```python
from build123d import *

# Parameters (mm, degrees)
CYLINDER412_R               = 1.5
CYLINDER412_DEPTH           = 60
CYLINDER410_R               = 1.5
CYLINDER410_DEPTH           = 60
CYLINDER410_PLACEMENT_ANGLE = 135
CYLINDER408_R               = 1.5
CYLINDER408_DEPTH           = 60
CYLINDER411_R               = 1.5
CYLINDER411_DEPTH           = 60
CYLINDER411_PLACEMENT_ANGLE = 225
CYLINDER414_R               = 1.5
CYLINDER414_DEPTH           = 60
CYLINDER407_R               = 1.5
CYLINDER407_DEPTH           = 60
CYLINDER407_PLACEMENT_ANGLE = 45
CYLINDER413_R               = 1.5
CYLINDER413_DEPTH           = 60
CYLINDER409_R               = 1.5
CYLINDER409_DEPTH           = 60
CYLINDER409_PLACEMENT_ANGLE = 45
COMPOUND307_PLACEMENT_ANGLE = 22.5
TUBE036_R                   = 46
TUBE036_R_2                 = 38
TUBE036_DEPTH               = 3


with BuildPart() as obj1:
    # Cylinder412 → Cylinder412 (new body)
    with BuildSketch(Plane(origin=(0, 41, -54), x_dir=(0, 1, 0), z_dir=(0, 0, 1))):
        Circle(CYLINDER412_R)
    extrude(amount=CYLINDER412_DEPTH)


with BuildPart() as obj2:
    # Cylinder410 → Cylinder410 (new body)
    with BuildSketch(Plane.XY):
        Circle(CYLINDER410_R)
    extrude(amount=CYLINDER410_DEPTH)


with BuildPart() as obj2_1:
    # Cylinder410 placement: moved
    add(obj2.part.moved(Location((-28.991378, 28.991378, -54))).rotate(Axis((-28.991378, 28.991378, -54), (0, 0, 1)), CYLINDER410_PLACEMENT_ANGLE))


with BuildPart() as obj3:
    # Cylinder408 → Cylinder408 (new body)
    with BuildSketch(Plane(origin=(-41, 0, -54), x_dir=(-1, 0, 0), z_dir=(0, 0, 1))):
        Circle(CYLINDER408_R)
    extrude(amount=CYLINDER408_DEPTH)


with BuildPart() as obj4:
    # Cylinder411 → Cylinder411 (new body)
    with BuildSketch(Plane.XY):
        Circle(CYLINDER411_R)
    extrude(amount=CYLINDER411_DEPTH)


with BuildPart() as obj4_1:
    # Cylinder411 placement: moved
    add(obj4.part.moved(Location((-28.991378, -28.991378, -54))).rotate(Axis((-28.991378, -28.991378, -54), (0, 0, 1)), CYLINDER411_PLACEMENT_ANGLE))


with BuildPart() as obj5:
    # Cylinder414 → Cylinder414 (new body)
    with BuildSketch(Plane(origin=(0, -41, -54), x_dir=(0, -1, 0), z_dir=(0, 0, 1))):
        Circle(CYLINDER414_R)
    extrude(amount=CYLINDER414_DEPTH)


with BuildPart() as obj6:
    # Cylinder407 → Cylinder407 (new body)
    with BuildSketch(Plane.XY):
        Circle(CYLINDER407_R)
    extrude(amount=CYLINDER407_DEPTH)


with BuildPart() as obj6_1:
    # Cylinder407 placement: moved
    add(obj6.part.moved(Location((28.991378, -28.991378, -54))).rotate(Axis((28.991378, -28.991378, -54), (0, 0, -1)), CYLINDER407_PLACEMENT_ANGLE))


with BuildPart() as obj7:
    # Cylinder413 → Cylinder413 (new body)
    with BuildSketch(Plane(origin=(41, 0, -54), x_dir=(1, 0, 0), z_dir=(0, 0, 1))):
        Circle(CYLINDER413_R)
    extrude(amount=CYLINDER413_DEPTH)


with BuildPart() as compound307:
    # Cylinder409 → Cylinder409 (new body)
    with BuildSketch(Plane.XY):
        Circle(CYLINDER409_R)
    extrude(amount=CYLINDER409_DEPTH)


with BuildPart() as compound307_1:
    # Cylinder409 placement: moved
    add(compound307.part.moved(Location((28.991378, 28.991378, -54))).rotate(Axis((28.991378, 28.991378, -54), (0, 0, 1)), CYLINDER409_PLACEMENT_ANGLE))

    # Compound307: union obj1, obj2, obj3, obj4, obj5, obj6, obj7
    add(obj1.part)
    add(obj2_1.part)
    add(obj3.part)
    add(obj4_1.part)
    add(obj5.part)
    add(obj6_1.part)
    add(obj7.part)


with BuildPart() as compound307_2:
    # Compound307 placement: moved
    add(compound307_1.part.rotate(Axis((0, 0, 0), (0, 0, 1)), COMPOUND307_PLACEMENT_ANGLE))


with BuildPart() as j_midi_motor_washer:
    # Tube036 → Tube036 (new body)
    with BuildSketch(Plane.XY.offset(-11)):
        Circle(TUBE036_R)
        Circle(TUBE036_R_2, mode=Mode.SUBTRACT)
    extrude(amount=TUBE036_DEPTH)

    # Cut162: cut Compound307
    add(compound307_2.part, mode=Mode.SUBTRACT)


solid = j_midi_motor_washer.part
```
Work out the finished part from the listing and answer in its coordinate system (mm). Coordinates: 2 decimals unless noted, no trailing zeros. Loops run counter-clockwise (first coordinate to the right, second up) from the corner with the lowest first, then second, coordinate; pieces in that order, holes last.
1) Section A-A (y = 0) is taken. Give the vertices of the cut face in (x, z), plus the area to 3 significant figures.
Results:
outline: (-46, -11) - (-38, -11) - (-38, -8) - (-46, -8) - close; (38, -11) - (46, -11) - (46, -8) - (38, -8) - close
area: 48.0 mm2
2) Consider probe 1 along X at (y, z) = (1, -9.6); probe 2 along Y at (x, z) = (13, -9.85); probe 3 along Y at (x, z) = (-23, -9.15). Determine where each line is inside the solid, lowest interval first.
Results:
probe 1: x = -45.99 to -37.99, 37.99 to 45.99
probe 2: y = -44.12 to -35.71, 35.71 to 44.12
probe 3: y = -39.84 to -30.25, 30.25 to 39.84
3) A flat-ended cylindrical pin translates along its axis: pin 1 (4 mm diameter, centred on x = 15.69, y = -37.88, fed in from -Z). Find the tip coordinate at first contact, or state that the pin passes through.
Results:
pin 1: stops at z = -11
4) Section C-C (z = -8.75) is taken. Give the number of separate pieces and of enclosed holes in the cut face, plus the area to 3 significant figures.
Results:
separate pieces: 1
enclosed holes: 9
area: 2,050 mm2
5) For a pull along Y with two mould halves and no side action, classify faces 1 (the cylindrical face through (-5.99, 45.61, -9.52)), 2 (the cylindrical face through (-14.33, -37.25, -9.52)), 3 (the flat face through (-7, 38, -11)) as +Y half, -Y half, draft (parallel to the pull), parting line (faces both ways), or undercut.
Results:
face 1: parting line
face 2: undercut
face 3: draft
